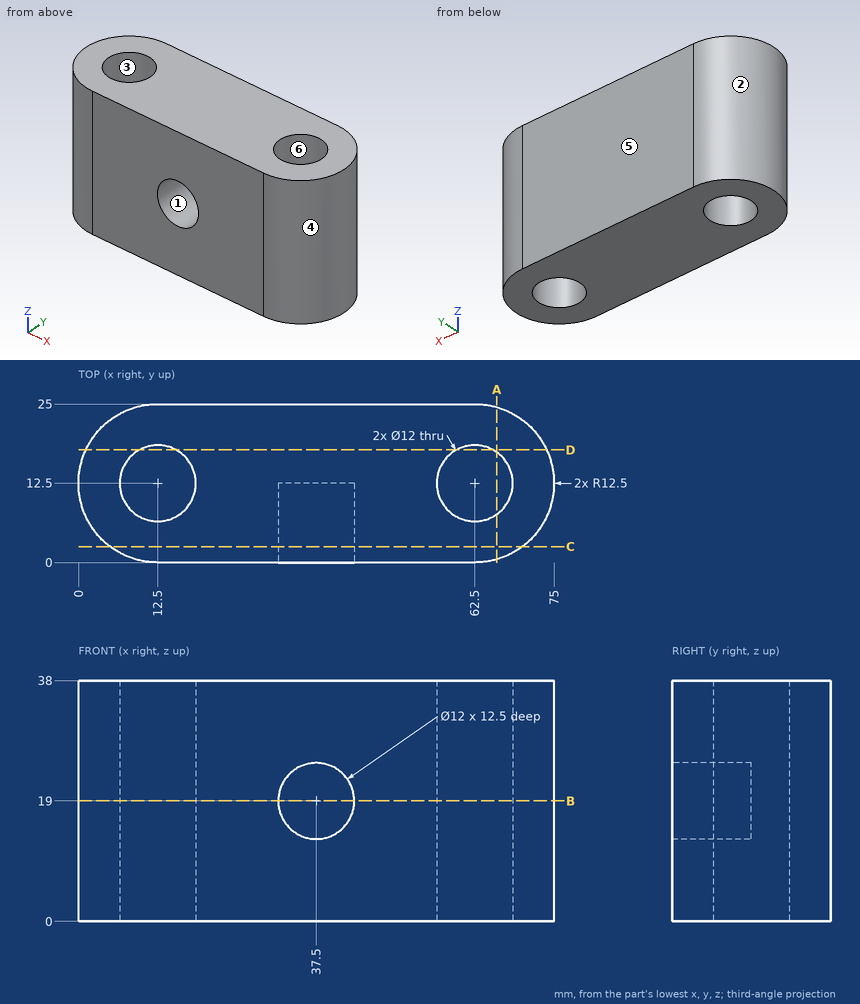
Can you work these out from the drawing? Everything is in mm from the part's minimum corner. A direction names the side the tool comes from. Round coordinates to 2 decimals unless told otherwise and drop trailing zeros. Write each loop counter-clockwise with the first axis right and the second up, starting at its lowest first coordinate (ties: lowest second). Pieces come first, ordered by that corner, then holes.
1. Suppose I cut it at C-C (y = 2.5). List the corners of the cut face in (x, z) for me, and give its area (3 significant figures).
2. For the marked faces 1 and 2, which set-ups out of +Z, -Z, +X, -X, +Y, -Y let a thin tool reach every point of the face, with its end or its side?
3. Suppose I cut it at A-A (x = 66). List the corners of the cut face in (y, z) for me.
4. Suppose I cut it at B-B (z = 19). List the corners of the cut face in (x, y) for me, and give its area (3 significant figures).
5. Suppose I cut it at D-D (y = 17.75). List the corners of the cut face in (x, z) for me, and give its area (3 significant figures).
6. If we mould it in two halves opening along X, with no side actions, what happens to the marked faces 3, 4, 5 and 6? For each: released by +X, released by -X, zero draft, split by the parting line, or undercut.
7. I need wall thicknesses on L1, parallel to Y at x = 62.5, z = 10; L2, parallel to X at y = 11.75, z = 27.5; L3, parallel to X at y = 9, z = 31.5. Which ranges of each line are inside material? Lowest first, please.
8. Will these pins go through, and if not, where does the flat tip stop? pin 1 Ø6 at (x, y) = (63.5, 5) entering from -Z; pin 2 Ø6 at (x, z) = (38, 20.5) entering from -Y; pin 3 Ø3 at (y, z) = (6.5, 9) entering from +X.
Answer sheet:
1. outline: (5, 0) - (70, 0) - (70, 38) - (5, 38) - close; hole circle Ø12 at (37.5, 19)
1. area: 2,360 mm2
2. face 1: -Y
2. face 2: +Z, -Z, -X
3. outline: (0.5, 0) - (7.63, 0) - (7.63, 38) - (0.5, 38) - close; (17.37, 0) - (24.5, 0) - (24.5, 38) - (17.37, 38) - close
4. outline: (12.5, 0) - (31.5, 0) - (31.5, 12.5) - (43.5, 12.5) - (43.5, 0) - (62.5, 0) arc R12.5 ccw to (62.5, 25) - (12.5, 25) arc R12.5 ccw to start; hole circle Ø12 at (12.5, 12.5); hole circle Ø12 at (62.5, 12.5)
4. area: 1,360 mm2
5. outline: (1.16, 0) - (9.6, 0) - (9.6, 38) - (1.16, 38) - close; (15.4, 0) - (59.6, 0) - (59.6, 38) - (15.4, 38) - close; (65.4, 0) - (73.84, 0) - (73.84, 38) - (65.4, 38) - close
5. area: 2,320 mm2
6. face 3: undercut
6. face 4: released by +X
6. face 5: zero draft
6. face 6: undercut
7. L1: y = 0 to 6.5, 18.5 to 25
7. L2: x = 0.02 to 6.55, 18.45 to 56.55, 68.45 to 74.98
7. L3: x = 0.5 to 7.63, 17.37 to 57.63, 67.37 to 74.5
8. pin 1: stops at z = 0
8. pin 2: stops at y = 12.5
8. pin 3: stops at x = 74.16
